The drawing under review shows one solid part. Ordinate dimensions are in mm from its lowest x, y, z. Round coordinates to 2 decimals unless told otherwise and drop trailing zeros. Use a Markdown table: item, result. Add a question column.
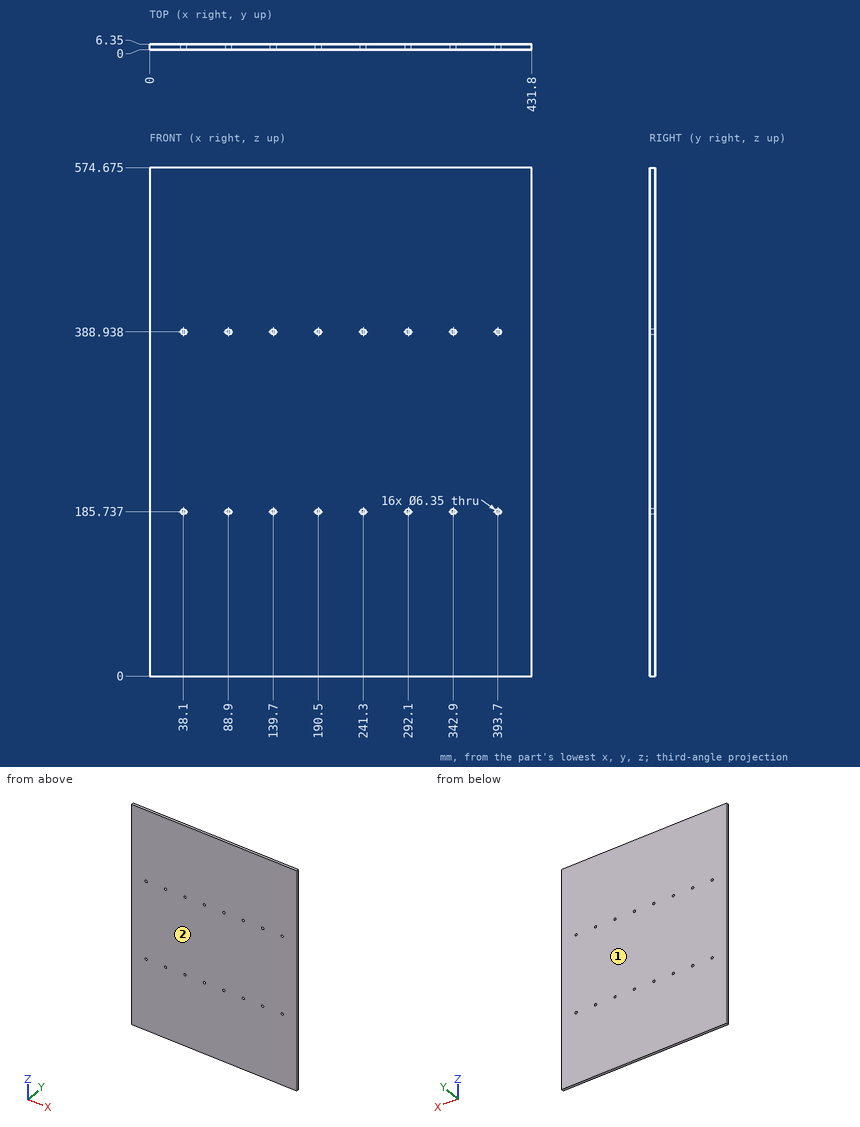
1. Mouldability with a two-part tool opening along Y and no side actions: class the marked faces 1 and 2 as +Y half, -Y half, draft (parallel to the pull), parting line (faces both ways), or undercut.
2. Insertion check: P1, Ø8.5, axis at x = 38.1, z = 185.74, coming from the -Y side; P2, Ø5, axis at x = 342.9, z = 185.74, coming from the +Y side. Each pin has a flat end and moves straight along its axis. Give the tip position at first contact, or say it passes through.
3. To check wall thickness, follow probe 1 along Z at (x, y) = (292.1, 3.25) (1 decimal). State the ranges of the line that lie inside material, in increasing order. Write a range as from..to.
Verdict:
| question | item | result |
|---|---|---|
| 1 | face 1 | +Y half |
| 1 | face 2 | -Y half |
| 2 | P1 | stops at y = 0 |
| 2 | P2 | passes through |
| 3 | probe 1 | z = 0..182.6, 188.9..385.8, 392.1..574.7 |
